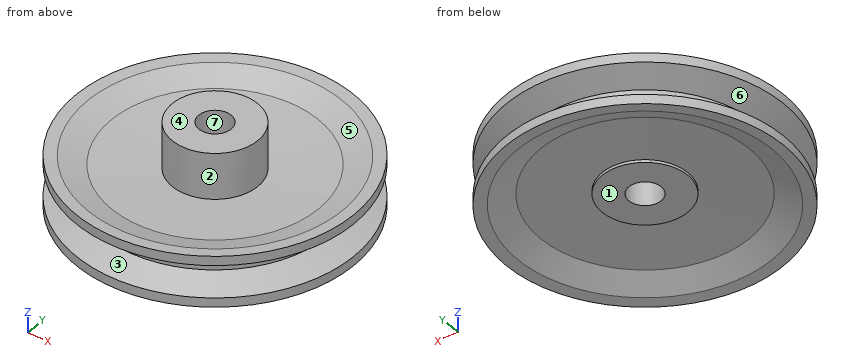
Autodesk Inventor part; units mm, degrees
ref_plane "YZ Plane" through (0, 0, 0) normal (1, 0, 0) x (0, 1, 0)
ref_plane "XZ Plane" through (0, 0, 0) normal (0, 1, 0) x (-1, 0, 0)
ref_plane "XY Plane" through (0, 0, 0) normal (0, 0, 1) x (1, 0, 0)
sketch "Sketch1" plane through (0, 0, 0) normal (0, 1, 0) x (-1, 0, 0)
  line L0 (0.0054, 10.9523) -> (60.0054, 10.9523)
  line L1 (60.0054, 10.9523) -> (60.0054, -11.0477)
  line L2 (60.0054, -11.0477) -> (0.0054, -11.0477)
  line L3 (0.0054, -11.0477) -> (0.0054, 10.9523)
  line L4 (60.0054, 10.9523) -> (60.0054, 6.9523)
  line L5 (60.0054, -11.0477) -> (60.0054, -7.0477)
  line L6 (60.0054, -0.0477) -> (49.0054, -0.0477)
  line L7 (49, 3) -> (49, -3)
  line L8 (49, 3) -> (55, 3) construction
  line L9 (49, -3) -> (60.0054, -7.0477)
  line L10 (49, 3) -> (60.0054, 6.9523)
  line L11 (60.0054, 10.9523) -> (45.0054, 10.9523)
  line L12 (60.0054, 10.9523) -> (55.0244, 10.5165)
  line L13 (60.0054, 10.9523) -> (65.0054, 10.9523) construction
  line L14 (55.0244, 10.5165) -> (44.6878, 6.7543)
  line L15 (55.0244, 10.5165) -> (66.0244, 10.5165) construction
  line L16 (60.0054, -11.0477) -> (55.0244, -10.612)
  line L17 (60.0054, -11.0477) -> (65.0054, -11.0477) construction
  line L18 (55.0244, -10.612) -> (45.055, -5.9631)
  line L19 (0, 4) -> (0, -4)
  line L20 (0, 4) -> (8, 4) construction
  line L21 (0, -4) -> (45.055, -5.9631)
  line L22 (44.6878, 6.7543) -> (0, 4)
  dimension "d1" = 60
  dimension "d2" = 22
  dimension "d3" = 4
  dimension "d4" = 4
  dimension "d5" = 11
  dimension "d6" = 6
  dimension "d7" = 90
  dimension "d8" = 15
  dimension "d9" = 5
  dimension "d10" = 175
  dimension "d11" = 11
  dimension "d12" = 160
  dimension "d13" = 5
  dimension "d14" = 175
  dimension "d15" = 11
  dimension "d16" = 160
  dimension "d17" = 8
  dimension "d18" = 90
revolve "Revolution1" add sketch "Sketch1" angle 360 about axis through (0, 0, 4) along (0, 0, -1) contours L22 L14 L12 L1 L10 L7 L9 L16 L18 L21 L3 | L3 L21 L19 L22
sketch "Sketch2" plane through (0, 0, 0) normal (0, 0, 1) x (1, 0, 0)
  circle A0 centre (0, 0) radius 18.5
  dimension "d20" = 37
extrude "Extrusion1" add sketch "Sketch2" along normal blind 25 and the other way blind 6
sketch "Sketch4" plane through (0, 0, 25) normal (0, 0, 1) x (1, 0, 0)
  circle A0 centre (0, 0) radius 7
  dimension "d25" = 14
extrude "Extrusion2" cut sketch "Sketch4" against normal blind 36
properties part number "bánh đà"
For this review, take the finished solid that the model builds, in its own axes (mm). Face numbers are marked on the shaded views. A direction names the side the tool comes from. Give positions to 0.01 mm unless a question says otherwise; leave off trailing zeros. Write each loop counter-clockwise with the first axis right and the second up, starting at its lowest first coordinate (ties: lowest second). Pieces come first, ordered by that corner, then holes. Notation, with made-up numbers: M -24.5,13.25 L 9.5,13.25 A23 ccw 9.5,43.25 Z; hole C 57,85 d2. An arc over 180 degrees is marked long. One line per item, written item: value.
1) For the marked faces 1, 2, 3 and 4, list the 3-axis set-ups (+Z, -Z, +X, -X, +Y, -Y) from which the entire face can be reached by the end or side of a thin tool; tool diameter is ignored.
Results are:
face 1: -Z
face 2: +Z
face 3: none
face 4: +Z, +X, -X, +Y, -Y
2) The part is to be moulded in two halves that separate along Z. For the marked faces 5, 6 and 7, say which applies: +Z half, -Z half, draft (parallel to the pull), parting line (faces both ways), or undercut.
Results are:
face 5: +Z half
face 6: undercut
face 7: draft
3) For P1, Ø18.5, axis at x = -6.5, y = 0, coming from the -Z side; P2, Ø5, axis at x = -10.5, z = 14.5, coming from the +Y side; P3, Ø10, axis at x = 14, z = 4, coming from the -Y side, all flat-tipped, find the tip position at first contact; note any pin that passes through.
Results are:
P1: stops at z = -6
P2: stops at y = 16.68
P3: stops at y = -59.17
4) For line 1 (Y direction, x = 0, z = 1.5); line 2 (Z direction, x = -10, y = 2.5); line 3 (X direction, y = -3.5, z = 22), list the stretches that pass through material, from the lowest coordinate up. Write a range as from..to.
Results are:
line 1: y = -49..-7, 7..49
line 2: z = -6..25
line 3: x = -18.17..-6.06, 6.06..18.17
5) Take a section at C-C, the plane z = 0. Write out the cut boundary in (x, y).
Results are:
outline: C 0,0 d98; hole C 0,0 d14
